```python
from build123d import *

# Parameters (mm, degrees)
SKETCH1_W               = 254
SKETCH1_H               = 3.175
BASE_FLANGE1_DEPTH      = 114.3
SKETCH6_R               = 12.7
CUT_EXTRUDE1_DEPTH      = 279.550840288
SKETCH7_R               = 2.286
CUT_EXTRUDE2_DEPTH      = 279.550840288
SKETCH9_R               = 3.556
CUT_EXTRUDE4_DEPTH      = 279.550840288
CUT_EXTRUDE6_DEPTH      = 279.550840288
CUT_EXTRUDE9_DEPTH      = 279.550840288
CUT_EXTRUDE9_DEPTH_BACK = 279.550840288
CUT_EXTRUDE10_DEPTH     = 221.768639368
FILLET1_R               = 50.8
CUT_EXTRUDE11_DEPTH     = 170.498049701
FILLET2_DEPTH           = 3.175


with BuildPart() as part:
    # Base-Flange1: sheet metal written as solids
    # Sketch1 → Base-Flange1 (new, symmetric)
    with BuildSketch(Plane.XY):
        with Locations((-127, 1.5875)):
            Rectangle(SKETCH1_W, SKETCH1_H)
    extrude(amount=BASE_FLANGE1_DEPTH, both=True)

    # Sketch6 → Cut-Extrude1 (cut, through all)
    with BuildSketch(Plane.XZ):
        with Locations(Location((-76.2, 82.55, 0), (0, 0, 270))):
            Circle(SKETCH6_R)
    extrude(amount=-CUT_EXTRUDE1_DEPTH, mode=Mode.SUBTRACT)

    # Sketch7 → Cut-Extrude2 (cut, through all)
    with BuildSketch(Plane.XZ):
        with Locations(Location((-43.18, 81.326566426, 0), (0, 0, 270))):
            Circle(SKETCH7_R)
        with Locations(Location((-109.22, 81.326566426, 0), (0, 0, 90))):
            Circle(SKETCH7_R)
        with Locations(Location((-76.2, 44.069, 0), (0, 0, 270))):
            Circle(SKETCH7_R)
    extrude(amount=-CUT_EXTRUDE2_DEPTH, mode=Mode.SUBTRACT)

    # Sketch9 → Cut-Extrude4 (cut, through all)
    with BuildSketch(Plane(origin=(0, 3.175, 0), x_dir=(1, 0, 0), z_dir=(0, 1, 0))):
        with Locations(Location((-12.7, 36.5125, 0), (0, 0, 180))):
            Circle(SKETCH9_R)
        with Locations((-12.7, 101.6)):
            Circle(SKETCH9_R)
        with Locations(Location((-12.7, -28.575, 0), (0, 0, 180))):
            Circle(SKETCH9_R)
        with Locations(Location((-88.9, 101.6, 0), (0, 0, 180))):
            Circle(SKETCH9_R)
    extrude(amount=-CUT_EXTRUDE4_DEPTH, mode=Mode.SUBTRACT)

    # Sketch15 → Cut-Extrude6 (cut, through all)
    with BuildSketch(Plane.XZ):
        Polygon((-101.6, -114.3), (-254, 38.1), (-254, -114.3), align=None)
    extrude(amount=-CUT_EXTRUDE6_DEPTH, mode=Mode.SUBTRACT)

    # Sketch17 → Cut-Extrude9 (cut, two sides: drawn at the far end of the back side and taken through both)
    with BuildSketch(Plane.XZ.offset(-CUT_EXTRUDE9_DEPTH_BACK)):
        with BuildLine():
            Line((-254, 114.3), (-254, 38.1))
            Line((-254, 38.1), (-159.5751337, -56.3248663))
            ThreePointArc((-159.5751337, -56.3248663), (-181.24151223, 52.599374135), (-88.9, 114.3))
            Line((-88.9, 114.3), (-254, 114.3))
        make_face()
    extrude(amount=CUT_EXTRUDE9_DEPTH + CUT_EXTRUDE9_DEPTH_BACK, mode=Mode.SUBTRACT)

    # Sketch18 → Cut-Extrude10 (cut, through all)
    with BuildSketch(Plane.XZ):
        with BuildLine():
            Line((-101.6, -114.3), (-101.6, -88.9))
            Line((-101.6, -88.9), (-52.208591334, -39.508591334))
            ThreePointArc((-52.208591334, -39.508591334), (-48.488847455, -30.528335213), (-52.208591334, -21.548079092))
            add(Edge.make_bspline(
                [(-106.256088924, 112.781538976), (-137.236150888, 107.318918188), (-113.262137977, 5.562411407), (-77.644814764, 3.888144338), (-52.208591334, -21.548079092)],
                knots=[0, 0, 0, 0, 0.537792704, 1, 1, 1, 1], degree=3))
            ThreePointArc((-106.256088924, 112.781538976), (-184.223754204, 44.405731651), (-159.5751337, -56.3248663))
            Line((-159.5751337, -56.3248663), (-101.6, -114.3))
        make_face()
    extrude(amount=-CUT_EXTRUDE10_DEPTH, mode=Mode.SUBTRACT)

    # Fillet1
    fillet1_edges = [part.edges().sort_by_distance(p)[0] for p in [
        (0, 1.5875, 114.3),
    ]]
    fillet(fillet1_edges, radius=FILLET1_R)

    # Sketch19 → Cut-Extrude11 (cut, through all)
    with BuildSketch(Plane(origin=(0, 3.175, 0), x_dir=(1, 0, 0), z_dir=(0, 1, 0))):
        with BuildLine():
            Line((-68.309231637, 88.9), (-31.75, 88.9))
            ThreePointArc((-31.75, 88.9), (-27.259871939, 87.040128061), (-25.4, 82.55))
            Line((-25.4, 82.55), (-25.4, 45.990768363))
            ThreePointArc((-25.4, 45.990768363), (-29.319960204, 40.124133332), (-36.240128061, 41.500640303))
            Line((-36.240128061, 41.500640303), (-72.799359697, 78.059871939))
            ThreePointArc((-72.799359697, 78.059871939), (-74.175866668, 84.980039796), (-68.309231637, 88.9))
        make_face()
        with BuildLine():
            Line((-25.4, 5.183084731), (-25.4, -63.31046263))
            ThreePointArc((-25.4, -63.31046263), (-28.690493445, -68.874806225), (-35.151785714, -68.672398284))
            ThreePointArc((-35.151785714, -68.672398284), (-39.759262533, -66.736201414), (-44.747192121, -66.422737896))
            ThreePointArc((-44.747192121, -66.422737896), (-47.9893887, -65.910636081), (-50.542713816, -63.847963596))
            ThreePointArc((-50.542713816, -63.847963596), (-54.493856691, -59.378771231), (-59.211239435, -55.727537129))
            ThreePointArc((-59.211239435, -55.727537129), (-61.771128872, -52.560544764), (-61.88090181, -48.489817008))
            ThreePointArc((-61.88090181, -48.489817008), (-61.530034533, -41.007577259), (-64.844174471, -34.290174786))
            Line((-64.844174471, -34.290174786), (-75.613232293, -21.784424959))
            ThreePointArc((-75.613232293, -21.784424959), (-77.094715661, -16.793975806), (-74.346704518, -12.372685217))
            add(Edge.make_bspline(
                [(-43.228335213, 12.567822971), (-46.917497652, 8.878660532), (-50.456440758, 5.648495964), (-57.219614246, -0.085464925), (-60.443504999, -2.588941631), (-66.531496779, -7.059997253), (-69.394290936, -9.027669237), (-72.834328708, -11.354789552), (-73.599593433, -11.869910022), (-74.346704518, -12.372685217)],
                knots=[0, 0, 0, 0, 0.0625, 0.0625, 0.125, 0.125, 0.1875, 0.1875, 0.205929014, 0.205929014, 0.205929014, 0.205929014], degree=3))
            ThreePointArc((-43.228335213, 12.567822971), (-31.847005437, 14.831710221), (-25.4, 5.183084731))
        make_face()
        with BuildLine():
            ThreePointArc((-110.360018807, -66.383991242), (-107.147438621, -66.484575814), (-104.030197179, -67.267898542))
            ThreePointArc((-104.030197179, -67.267898542), (-99.340434929, -60.811031043), (-93.188760565, -55.727537129))
            ThreePointArc((-93.188760565, -55.727537129), (-90.628871128, -52.560544764), (-90.51909819, -48.489817008))
            ThreePointArc((-90.51909819, -48.489817008), (-90.463817251, -39.472945885), (-85.244463491, -32.12003033))
            ThreePointArc((-85.244463491, -32.12003033), (-84.622720301, -25.604510261), (-91.167480683, -25.536115004))
            add(Edge.make_bspline(
                [(-91.167480683, -25.536115004), (-92.635934993, -27.101357134), (-94.055170685, -28.817008687), (-96.262497765, -31.913028022), (-97.045227937, -33.09572145), (-98.628898545, -35.6878173), (-99.428995475, -37.095537018), (-101.805342608, -41.586869819), (-103.35622482, -44.937897773), (-106.205005263, -52.031513868), (-107.504026121, -55.775168297), (-109.265538459, -61.831529556), (-109.854670713, -64.117538163), (-110.360018807, -66.383991242)],
                knots=[0.380798959, 0.380798959, 0.380798959, 0.380798959, 0.4375, 0.4375, 0.46875, 0.46875, 0.5, 0.5, 0.5625, 0.5625, 0.625, 0.625, 0.662483442, 0.662483442, 0.662483442, 0.662483442], degree=3))
        make_face()
    extrude(amount=-CUT_EXTRUDE11_DEPTH, mode=Mode.SUBTRACT)

    # Fillet2: read off the stored shape, not the designer's step
    # Fillet2 outline → Fillet2 (add)
    with BuildSketch(Plane(origin=(0, 0, 0), x_dir=(1.0, 1.1573850035061633e-12, 0), z_dir=(-1.1573850035061633e-12, 1.0, 0))):
        with BuildLine():
            ThreePointArc((-104.030197179, -67.267898542), (-103.374185767, -66.129703781), (-102.671651197, -65.019621142))
            add(Edge.make_bspline(
                [(-102.671651197, -65.019621142), (-103.429510547, -66.164022442), (-104.780608937, -66.91555764), (-106.42610863, -66.603307038)],
                knots=[0, 0, 0, 0, 0.430480656, 0.430480656, 0.430480656, 0.430480656], degree=3, weights=[1, 0.75936345, 0.62231628, 0.58885849]))
            ThreePointArc((-106.42610863, -66.603307038), (-105.214346034, -66.885827792), (-104.030197179, -67.267898542))
        make_face()
        with BuildLine():
            ThreePointArc((-110.360018807, -66.383991242), (-108.385824678, -66.363801056), (-106.42610863, -66.603307038))
            add(Edge.make_bspline(
                [(-106.42610863, -66.603307038), (-108.913766663, -66.131248173), (-109.817041103, -63.994539841), (-109.296016182, -62.039816736)],
                knots=[0.430480656, 0.430480656, 0.430480656, 0.430480656, 1, 1, 1, 1], degree=3, weights=[0.58885849, 0.544594344, 0.681641514, 1]))
            add(Edge.make_bspline(
                [(-109.296016182, -62.039816736), (-109.682496439, -63.489770196), (-110.038242372, -64.940845021), (-110.360018807, -66.383991242)],
                knots=[0.638616154, 0.638616154, 0.638616154, 0.638616154, 0.662483442, 0.662483442, 0.662483442, 0.662483442], degree=3))
        make_face()
    extrude(amount=FILLET2_DEPTH)


solid = part.part
```
Input: part model. Units: mm. Frame: model coordinates. Round coordinates to 2 decimals unless told otherwise and drop trailing zeros. Loops run counter-clockwise (first coordinate to the right, second up) from the corner with the lowest first, then second, coordinate; pieces in that order, holes last. Notation, with made-up numbers: M -31.75,60.5 L 23.25,60.5 A18 cw 23.25,87.5 Z; hole C -31.75,5.25 d9. An arc over 180 degrees is marked long. Answer in a Markdown table with one row per item. Add a question column.
1. Section A-A (z = -85.5). Output: boundary loops of the cut face in (x, y) (3 decimals), and give its area (3 significant figures).
2. Section D-D (y = 2.1). Give the number of separate pieces and of enclosed holes in the cut face, and give its area (3 significant figures).
3. Section C-C (z = -61). Output: boundary loops of the cut face in (x, y) (3 decimals).
4. Ray query, probe 1 along Z at (x, y) = (-12.7, 1.5); probe 2 along Z at (x, y) = (-12, 2); probe 3 along X at (y, z) = (0.3, 59). Return the intervals inside material, ascending.
5. Mould query, pull axis X, two halves, no side actions, for faces 1 (the face through (-15.276, 1.61, 99.814)), 2 (the face through (-14.612, 1.61, -33.514)), 3 (the face through (-77.3, 1.6, -64.6)), 4 (the face through (-92.185, 1.61, -102.962)). Classes: released by +X, released by -X, zero draft, split by the parting line, or undercut.
6. Contact query for flat-ended pins moving along their axis: pin 1 (1.6 mm diameter, centred on x = -48, y = 1, fed in from +Z); pin 2 (1.5 mm diameter, centred on x = -103, y = 2.5, fed in from -Z); pin 3 (1 mm diameter, centred on x = -33.5, y = 3, fed in from +Z). Output: stop coordinate, or through.
7. Section B-B (x = -12.7). Output: boundary loops of the cut face in (y, z) (1 decimal), and give its area (3 significant figures).
Values follow:
| question | item | result |
|---|---|---|
| 1 | outline | M -98.2,0 L -73.932,0 L -73.932,3.175 L -98.2,3.175 Z; M -26.127,0 L 0,0 L 0,3.175 L -26.127,3.175 Z |
| 1 | area | 160 mm^2 |
| 2 | separate pieces | 1 |
| 2 | enclosed holes | 11 |
| 2 | area | 15,400 mm^2 |
| 3 | outline | M -73.7,0 L -55.739,0 L -55.739,3.175 L -73.7,3.175 Z; M -25.4,0 L 0,0 L 0,3.175 L -25.4,3.175 Z |
| 4 | probe 1 | -114.3 to -105.16, -98.04 to -40.07, -32.96 to 25.02, 32.13 to 97.1 |
| 4 | probe 2 | -114.3 to -105.09, -98.11 to -40, -33.03 to 25.09, 32.06 to 96.29 |
| 4 | probe 3 | -121.63 to -108.44, -97.49 to -54.91, -25.4 to 0 |
| 5 | face 1 | released by +X |
| 5 | face 2 | undercut |
| 5 | face 3 | released by -X |
| 5 | face 4 | undercut |
| 6 | pin 1 | z = 114.26 |
| 6 | pin 2 | z = 18.88 |
| 6 | pin 3 | z = 111.44 |
| 7 | outline | M 0,-114.3 L 3.2,-114.3 L 3.2,-105.2 L 0,-105.2 Z; M 0,-98 L 3.2,-98 L 3.2,-40.1 L 0,-40.1 Z; M 0,-33 L 3.2,-33 L 3.2,25 L 0,25 Z; M 0,32.1 L 3.2,32.1 L 3.2,97.1 L 0,97.1 Z |
| 7 | area | 603 mm^2 |
